The listing builds one solid part. Answer for the finished solid, in the listing's coordinates (mm). A direction names the side the tool comes from. Round coordinates to 2 decimals unless told otherwise and drop trailing zeros. Order: outer loops, then holes, each group sorted by start corner. A loop starts at its lowest first (then second) coordinate and runs counter-clockwise, first axis right, second up. Notation, with made-up numbers: (-37.5, 39) - (1.5, 39) arc R14 cw to (1.5, 52) - close; hole circle Ø9 at (21.5, 52.25). An arc over 180 degrees is marked (long way). Use CSV: the item, a comma, the result in double quotes. Start each with the question number.
Item 1: Flat-ended cylindrical pins translate along their axes: P1, Ø8, axis at x = 0.5, y = 10.5, coming from the +Z side; P2, Ø11, axis at x = 125, z = -48, coming from the +Y side. Find the tip coordinate at first contact, or state that the pin passes through.
Item 2: Find section A-A, the plane x = 125. Count the separate pieces of the cut face and the enclosed holes in it, plus the area to 3 significant figures.
Item 3: Find section C-C, the plane x = 5.5. Give the vertices of the cut face in (y, z).
Item 4: Find section B-B, the plane z = -58. Give the vertices of the cut face in (x, y).
Item 5: For faces 1 (the flat face through (-136.8, 6, -1)), 2 (the flat face through (-69, 7, -71.3)), 3 (the cylindrical face through (24.813, -0.345, 52.246)), determine the directions among +Z, -Z, +X, -X, +Y, -Y from which every point of the face is accessible in a straight line to the end or side of a thin tool.
Item 6: Straight lines are drawn through the part: line 1 along Z through (x, y) = (-87.5, 3); line 2 along X through (y, z) = (3, 14.5); line 3 along Z through (x, y) = (125, -0.15). For each, find the intervals that lie inside material, in ascending order. Write a range as [from, to].
Item 7: Determine the mould class of faces 4 (the flat face through (-137.5, 6, -1)), 5 (the flat face through (-70, 7, 71.3)), 6 (the cylindrical face through (-122.128, -0.345, -51.132)) for opening direction X: +X half, -X half, draft (parallel to the pull), parting line (faces both ways), or undercut.
```python
from build123d import *

# Parameters (mm, degrees)
SKETCH_1_W                         = 275
SKETCH_1_H                         = 144
SKETCH_1_R                         = 4.25
SM_BASE_FLANGE_1_DEPTH             = 0.7
SM_EDGE_FLANGE_1_STRIP_W           = 3.2
SM_EDGE_FLANGE_1_STRIP_H           = 0.7
SM_EDGE_FLANGE_1_STRIP_CUT_DEPTH   = 275
SM_EDGE_FLANGE_1_STRIP_2_W         = 3.2
SM_EDGE_FLANGE_1_STRIP_2_H         = 0.7
SM_EDGE_FLANGE_1_STRIP_CUT_2_DEPTH = 275
SM_EDGE_FLANGE_1_DEPTH             = 275
SM_EDGE_FLANGE_1_BEND_DEPTH        = 275
SKETCH_14_R                        = 3
CUT_EXTRUDE_1_DEPTH                = 10
SKETCH_15_R                        = 3
CUT_EXTRUDE_2_DEPTH                = 10
SKETCH_16_W                        = 3
SKETCH_16_H                        = 13.3
CUT_EXTRUDE_3_DEPTH                = 10
SKETCH_17_W                        = 3
SKETCH_17_H                        = 13.3
CUT_EXTRUDE_4_DEPTH                = 10
SM_EDGE_FLANGE_2_STRIP_W           = 3.2
SM_EDGE_FLANGE_2_STRIP_H           = 0.7
SM_EDGE_FLANGE_2_STRIP_CUT_DEPTH   = 142.2
SM_EDGE_FLANGE_2_STRIP_2_W         = 3.2
SM_EDGE_FLANGE_2_STRIP_2_H         = 0.7
SM_EDGE_FLANGE_2_STRIP_CUT_2_DEPTH = 142.2
SM_EDGE_FLANGE_2_DEPTH             = 142.2
SM_EDGE_FLANGE_2_BEND_DEPTH        = 142.2


# Sheet-metal steps are written as plain solids
with BuildPart() as part:
    # Sketch 1 → 基体-法兰1 (new body)
    with BuildSketch(Plane(origin=(0, 0, 0), x_dir=(1, 0, 0), z_dir=(0, 1, 0))):
        Rectangle(SKETCH_1_W, SKETCH_1_H)
        with Locations(Location((-125, -48, 0), (0, 0, 270))):
            Circle(SKETCH_1_R, mode=Mode.SUBTRACT)
        with Locations(Location((-125, -24, 0), (0, 0, 270))):
            Circle(SKETCH_1_R, mode=Mode.SUBTRACT)
        with Locations(Location((-125, 0, 0), (0, 0, 270))):
            Circle(SKETCH_1_R, mode=Mode.SUBTRACT)
        with Locations(Location((-125, 24, 0), (0, 0, 270))):
            Circle(SKETCH_1_R, mode=Mode.SUBTRACT)
        with Locations(Location((-125, 48, 0), (0, 0, 270))):
            Circle(SKETCH_1_R, mode=Mode.SUBTRACT)
        with Locations(Location((-75, -48, 0), (0, 0, 90))):
            Circle(SKETCH_1_R, mode=Mode.SUBTRACT)
        with Locations(Location((-75, -24, 0), (0, 0, 90))):
            Circle(SKETCH_1_R, mode=Mode.SUBTRACT)
        with Locations(Location((-75, 0, 0), (0, 0, 90))):
            Circle(SKETCH_1_R, mode=Mode.SUBTRACT)
        with Locations(Location((-75, 24, 0), (0, 0, 90))):
            Circle(SKETCH_1_R, mode=Mode.SUBTRACT)
        with Locations(Location((-75, 48, 0), (0, 0, 90))):
            Circle(SKETCH_1_R, mode=Mode.SUBTRACT)
        with Locations(Location((-25, -48, 0), (0, 0, 270))):
            Circle(SKETCH_1_R, mode=Mode.SUBTRACT)
        with Locations(Location((-25, -24, 0), (0, 0, 270))):
            Circle(SKETCH_1_R, mode=Mode.SUBTRACT)
        with Locations(Location((-25, 0, 0), (0, 0, 270))):
            Circle(SKETCH_1_R, mode=Mode.SUBTRACT)
        with Locations(Location((-25, 24, 0), (0, 0, 270))):
            Circle(SKETCH_1_R, mode=Mode.SUBTRACT)
        with Locations(Location((-25, 48, 0), (0, 0, 270))):
            Circle(SKETCH_1_R, mode=Mode.SUBTRACT)
        with Locations(Location((25, -48, 0), (0, 0, 90))):
            Circle(SKETCH_1_R, mode=Mode.SUBTRACT)
        with Locations(Location((25, -24, 0), (0, 0, 90))):
            Circle(SKETCH_1_R, mode=Mode.SUBTRACT)
        with Locations(Location((25, 0, 0), (0, 0, 90))):
            Circle(SKETCH_1_R, mode=Mode.SUBTRACT)
        with Locations(Location((25, 24, 0), (0, 0, 90))):
            Circle(SKETCH_1_R, mode=Mode.SUBTRACT)
        with Locations(Location((25, 48, 0), (0, 0, 90))):
            Circle(SKETCH_1_R, mode=Mode.SUBTRACT)
        with Locations(Location((75, 48, 0), (0, 0, 270))):
            Circle(SKETCH_1_R, mode=Mode.SUBTRACT)
        with Locations(Location((75, 24, 0), (0, 0, 270))):
            Circle(SKETCH_1_R, mode=Mode.SUBTRACT)
        with Locations(Location((75, 0, 0), (0, 0, 270))):
            Circle(SKETCH_1_R, mode=Mode.SUBTRACT)
        with Locations(Location((75, -24, 0), (0, 0, 270))):
            Circle(SKETCH_1_R, mode=Mode.SUBTRACT)
        with Locations(Location((75, -48, 0), (0, 0, 270))):
            Circle(SKETCH_1_R, mode=Mode.SUBTRACT)
        with Locations(Location((125, -48, 0), (0, 0, 90))):
            Circle(SKETCH_1_R, mode=Mode.SUBTRACT)
        with Locations(Location((125, -24, 0), (0, 0, 90))):
            Circle(SKETCH_1_R, mode=Mode.SUBTRACT)
        with Locations(Location((125, 0, 0), (0, 0, 90))):
            Circle(SKETCH_1_R, mode=Mode.SUBTRACT)
        with Locations(Location((125, 24, 0), (0, 0, 90))):
            Circle(SKETCH_1_R, mode=Mode.SUBTRACT)
        with Locations(Location((125, 48, 0), (0, 0, 90))):
            Circle(SKETCH_1_R, mode=Mode.SUBTRACT)
    extrude(amount=-SM_BASE_FLANGE_1_DEPTH)

    # 边线-法兰1 strip (across the edge) → 边线-法兰1 strip cut (cut)
    with BuildSketch(Plane(origin=(-137.5, 0, 72), x_dir=(0, 0, -1), z_dir=(1, 0, 0))):
        with Locations((-0.7, -0.35)):
            Rectangle(SM_EDGE_FLANGE_1_STRIP_W, SM_EDGE_FLANGE_1_STRIP_H)
    extrude(amount=SM_EDGE_FLANGE_1_STRIP_CUT_DEPTH, mode=Mode.SUBTRACT)

    # 边线-法兰1 strip 2 (across the edge) → 边线-法兰1 strip cut 2 (cut)
    with BuildSketch(Plane(origin=(137.5, 0, -72), x_dir=(0, 0, 1), z_dir=(-1, 0, 0))):
        with Locations((-0.7, -0.35)):
            Rectangle(SM_EDGE_FLANGE_1_STRIP_2_W, SM_EDGE_FLANGE_1_STRIP_2_H)
    extrude(amount=SM_EDGE_FLANGE_1_STRIP_CUT_2_DEPTH, mode=Mode.SUBTRACT)

    # 边线-法兰1 section (across the edge) → 边线-法兰1 (add)
    with BuildSketch(Plane(origin=(-137.5, 0, 72), x_dir=(0, 0, -1), z_dir=(1, 0, 0))):
        with BuildLine():
            Line((0, 0.2), (0, 13.3))
            Line((0, 13.3), (0.7, 13.3))
            Line((0.7, 13.3), (0.7, 0.2))
            ThreePointArc((0.7, 0.2), (0.758578644, 0.058578644), (0.9, 0))
            Line((0.9, 0), (0.9, -0.7))
            ThreePointArc((0.9, -0.7), (0.263603897, -0.436396103), (0, 0.2))
        make_face()
    extrude(amount=SM_EDGE_FLANGE_1_DEPTH)

    # 边线-法兰1 section 2 (across the edge) → 边线-法兰1 bend (add)
    with BuildSketch(Plane(origin=(137.5, 0, -72), x_dir=(0, 0, 1), z_dir=(-1, 0, 0))):
        with BuildLine():
            Line((0, 0.2), (0, 13.3))
            Line((0, 13.3), (0.7, 13.3))
            Line((0.7, 13.3), (0.7, 0.2))
            ThreePointArc((0.7, 0.2), (0.758578644, 0.058578644), (0.9, 0))
            Line((0.9, 0), (0.9, -0.7))
            ThreePointArc((0.9, -0.7), (0.263603897, -0.436396103), (0, 0.2))
        make_face()
    extrude(amount=SM_EDGE_FLANGE_1_BEND_DEPTH)

    # 草图14 → 切除-拉伸1 (cut)
    with BuildSketch(Plane(origin=(0, 0, 71.3), x_dir=(-1, 0, 0), z_dir=(0, 0, -1))):
        with Locations((-132, 7.8)):
            Circle(SKETCH_14_R)
        with Locations((0, 7.8)):
            Circle(SKETCH_14_R)
        with Locations((132, 7.8)):
            Circle(SKETCH_14_R)
    extrude(amount=-CUT_EXTRUDE_1_DEPTH, mode=Mode.SUBTRACT)

    # 草图15 → 切除-拉伸2 (cut)
    with BuildSketch(Plane(origin=(0, 0, -72), x_dir=(-1, 0, 0), z_dir=(0, 0, -1))):
        with Locations((-132, 7.8)):
            Circle(SKETCH_15_R)
        with Locations((0, 7.8)):
            Circle(SKETCH_15_R)
        with Locations((132, 7.8)):
            Circle(SKETCH_15_R)
    extrude(amount=-CUT_EXTRUDE_2_DEPTH, mode=Mode.SUBTRACT)

    # 草图16 → 切除-拉伸3 (cut)
    with BuildSketch(Plane(origin=(0, 0, -72), x_dir=(-1, 0, 0), z_dir=(0, 0, -1))):
        with Locations((0, 6.65)):
            Rectangle(SKETCH_16_W, SKETCH_16_H)
    extrude(amount=-CUT_EXTRUDE_3_DEPTH, mode=Mode.SUBTRACT)

    # 草图17 → 切除-拉伸4 (cut)
    with BuildSketch(Plane.XY.offset(72)):
        with Locations((0, 6.65)):
            Rectangle(SKETCH_17_W, SKETCH_17_H)
    extrude(amount=-CUT_EXTRUDE_4_DEPTH, mode=Mode.SUBTRACT)

    # 边线-法兰2 strip (across the edge) → 边线-法兰2 strip cut (cut)
    with BuildSketch(Plane(origin=(-137.5, 0, -71.1), x_dir=(1, 0, 0), z_dir=(0, 0, 1))):
        with Locations((-0.7, -0.35)):
            Rectangle(SM_EDGE_FLANGE_2_STRIP_W, SM_EDGE_FLANGE_2_STRIP_H)
    extrude(amount=SM_EDGE_FLANGE_2_STRIP_CUT_DEPTH, mode=Mode.SUBTRACT)

    # 边线-法兰2 strip 2 (across the edge) → 边线-法兰2 strip cut 2 (cut)
    with BuildSketch(Plane(origin=(137.5, 0, 71.1), x_dir=(-1, 0, 0), z_dir=(0, 0, -1))):
        with Locations((-0.7, -0.35)):
            Rectangle(SM_EDGE_FLANGE_2_STRIP_2_W, SM_EDGE_FLANGE_2_STRIP_2_H)
    extrude(amount=SM_EDGE_FLANGE_2_STRIP_CUT_2_DEPTH, mode=Mode.SUBTRACT)

    # 边线-法兰2 section (across the edge) → 边线-法兰2 (add)
    with BuildSketch(Plane(origin=(-137.5, 0, -71.1), x_dir=(1, 0, 0), z_dir=(0, 0, 1))):
        with BuildLine():
            Line((0, 0.2), (0, 11.8))
            Line((0, 11.8), (0.7, 11.8))
            Line((0.7, 11.8), (0.7, 0.2))
            ThreePointArc((0.7, 0.2), (0.758578644, 0.058578644), (0.9, 0))
            Line((0.9, 0), (0.9, -0.7))
            ThreePointArc((0.9, -0.7), (0.263603897, -0.436396103), (0, 0.2))
        make_face()
    extrude(amount=SM_EDGE_FLANGE_2_DEPTH)

    # 边线-法兰2 section 2 (across the edge) → 边线-法兰2 bend (add)
    with BuildSketch(Plane(origin=(137.5, 0, 71.1), x_dir=(-1, 0, 0), z_dir=(0, 0, -1))):
        with BuildLine():
            Line((0, 0.2), (0, 11.8))
            Line((0, 11.8), (0.7, 11.8))
            Line((0.7, 11.8), (0.7, 0.2))
            ThreePointArc((0.7, 0.2), (0.758578644, 0.058578644), (0.9, 0))
            Line((0.9, 0), (0.9, -0.7))
            ThreePointArc((0.9, -0.7), (0.263603897, -0.436396103), (0, 0.2))
        make_face()
    extrude(amount=SM_EDGE_FLANGE_2_BEND_DEPTH)


solid = part.part
```
Worked out:
1,P1,"stops at z = 72"
1,P2,"stops at y = 0"
2,separate pieces,"6"
2,enclosed holes,"0"
2,area,"89.3 mm²"
3,outline,"(-0.7, -71.1) arc R0.9 ccw to (0.2, -72) - (13.3, -72) - (13.3, -71.3) - (0.2, -71.3) arc R0.2 cw to (0, -71.1) - (0, 71.1) arc R0.2 cw to (0.2, 71.3) - (13.3, 71.3) - (13.3, 72) - (0.2, 72) arc R0.9 ccw to (-0.7, 71.1) - close"
4,outline,"(-137.5, 0.2) arc R0.9 ccw to (-136.6, -0.7) - (136.6, -0.7) arc R0.9 ccw to (137.5, 0.2) - (137.5, 11.8) - (136.8, 11.8) - (136.8, 0.2) arc R0.2 cw to (136.6, 0) - (-136.6, 0) arc R0.2 cw to (-136.8, 0.2) - (-136.8, 11.8) - (-137.5, 11.8) - close"
5,face 1,"+Y"
5,face 2,"+X, -X, +Y"
5,face 3,"+Y, -Y"
6,line 1,"z = [-72, -71.3], [71.3, 72]"
6,line 2,"x = [-137.5, -136.8], [136.8, 137.5]"
6,line 3,"z = [-71.93, -52.25], [-43.75, -28.25], [-19.75, -4.25], [4.25, 19.75], [28.25, 43.75], [52.25, 71.93]"
7,face 4,"-X half"
7,face 5,"draft"
7,face 6,"undercut"
